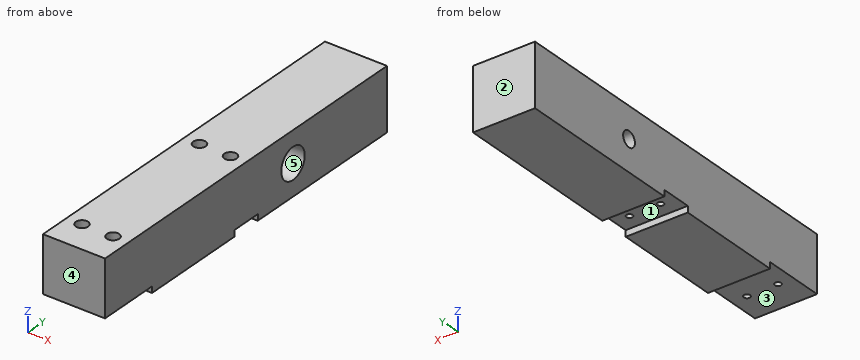
from build123d import *

# Parameters (mm, degrees)
SKETCH1_W           = 20
SKETCH1_H           = 120
SKETCH1_R           = 2.5
BOSS_EXTRUDE2_DEPTH = 20
SKETCH10_R          = 5
CUT_EXTRUDE1_DEPTH  = 10
SKETCH11_R          = 1
CUT_EXTRUDE2_DEPTH  = 21
SKETCH12_R          = 2
CUT_EXTRUDE3_DEPTH  = 5
SKETCH11_3_R        = 1
CUT_EXTRUDE4_DEPTH  = 21
SKETCH14_W          = 20
SKETCH14_H          = 10
SKETCH14_H_2        = 20
CUT_EXTRUDE6_DEPTH  = 2


with BuildPart() as part:
    # Sketch1 → Boss-Extrude2 (new body)
    with BuildSketch(Plane(origin=(0, 0, 0), x_dir=(0, 0, -1), z_dir=(1, 0, 0))):
        with Locations((10, 60)):
            Rectangle(SKETCH1_W, SKETCH1_H)
        with Locations((10, 80)):
            Circle(SKETCH1_R, mode=Mode.SUBTRACT)
    extrude(amount=-BOSS_EXTRUDE2_DEPTH)

    # Sketch10 → Cut-Extrude1 (cut)
    with BuildSketch(Plane(origin=(0, 0, 0), x_dir=(0, 0, -1), z_dir=(1, 0, 0))):
        with Locations((10, 80)):
            Circle(SKETCH10_R)
    extrude(amount=-CUT_EXTRUDE1_DEPTH, mode=Mode.SUBTRACT)

    # Sketch11 → Cut-Extrude2 (cut, through all)
    with BuildSketch(Plane.XY):
        with Locations((-15, 10)):
            Circle(SKETCH11_R)
        with Locations((-5, 10)):
            Circle(SKETCH11_R)
    extrude(amount=-CUT_EXTRUDE2_DEPTH, mode=Mode.SUBTRACT)

    # Sketch12 → Cut-Extrude3 (cut)
    with BuildSketch(Plane.XY):
        with Locations((-15, 10)):
            Circle(SKETCH12_R)
        with Locations((-5, 10)):
            Circle(SKETCH12_R)
        with Locations((-15, 60)):
            Circle(SKETCH12_R)
        with Locations((-5, 60)):
            Circle(SKETCH12_R)
    extrude(amount=-CUT_EXTRUDE3_DEPTH, mode=Mode.SUBTRACT)

    # Sketch11<3> → Cut-Extrude4 (cut, through all)
    with BuildSketch(Plane.XY):
        with Locations((-15, 60)):
            Circle(SKETCH11_3_R)
        with Locations((-5, 60)):
            Circle(SKETCH11_3_R)
    extrude(amount=-CUT_EXTRUDE4_DEPTH, mode=Mode.SUBTRACT)

    # Sketch14 → Cut-Extrude6 (cut)
    with BuildSketch(Plane(origin=(0, 0, -20), x_dir=(-1, 0, 0), z_dir=(0, 0, -1))):
        with Locations((10, 60)):
            Rectangle(SKETCH14_W, SKETCH14_H)
        with Locations((10, 10)):
            Rectangle(SKETCH14_W, SKETCH14_H_2)
    extrude(amount=-CUT_EXTRUDE6_DEPTH, mode=Mode.SUBTRACT)


solid = part.part
Design review of the part built by this model. Coordinates are the model's own, in mm. Face numbers are marked on the shaded views. A direction names the side the tool comes from. Coordinates: 2 decimals unless noted, no trailing zeros. Write each loop counter-clockwise with the first axis right and the second up, starting at its lowest first coordinate (ties: lowest second). Pieces come first, ordered by that corner, then holes. Notation, with made-up numbers: (18, 37.5) - (46, 37.5) arc R8 cw to (46, 42.5) - close; hole circle Ø7 at (84, -11.5). An arc over 180 degrees is marked (long way). Use one line per item in the form item = value.
Q1. For probe 1 along Y at (x, z) = (-5, -3.1); probe 2 along Y at (x, z) = (-5, -9.75); probe 3 along Y at (x, z) = (-3.5, -19), list the stretches that pass through material, from the lowest coordinate up.
Taken from the geometry:
probe_1 = 0 to 8, 12 to 58, 62 to 120
probe_2 = 0 to 9, 11 to 59, 61 to 75.01, 84.99 to 120
probe_3 = 20 to 55, 65 to 120
Q2. The part is to be moulded in two halves that separate along Y. For the marked faces 1, 2 and 3, say which applies: +Y half, -Y half, draft (parallel to the pull), parting line (faces both ways), or undercut.
Taken from the geometry:
face_1 = undercut
face_2 = +Y half
face_3 = draft
Q3. Machinability: for the marked faces 4 and 5, which of the approach directions +Z, -Z, +X, -X, +Y, -Y give a long, thin tool a straight path to every point of the face, cutting with its end or side? Answer none if there is none.
Taken from the geometry:
face_4 = +Z, -Z, +X, -X, -Y
face_5 = +X
Q4. Consider section C-C (z = -10). Write out the cut boundary in (x, y).
Taken from the geometry:
outline = (-20, 0) - (0, 0) - (0, 75) - (-10, 75) - (-10, 77.5) - (-20, 77.5) - close; (-20, 82.5) - (-10, 82.5) - (-10, 85) - (0, 85) - (0, 120) - (-20, 120) - close; hole circle Ø2 at (-15, 10); hole circle Ø2 at (-15, 60); hole circle Ø2 at (-5, 10); hole circle Ø2 at (-5, 60)
Q5. Consider section A-A (x = -15). Write out the cut boundary in (y, z), plus the area to 3 significant figures.
Taken from the geometry:
outline = (0, -18) - (9, -18) - (9, -5) - (8, -5) - (8, 0) - (0, 0) - close; (11, -18) - (20, -18) - (20, -20) - (55, -20) - (55, -18) - (59, -18) - (59, -5) - (58, -5) - (58, 0) - (12, 0) - (12, -5) - (11, -5) - close; (61, -18) - (65, -18) - (65, -20) - (120, -20) - (120, 0) - (62, 0) - (62, -5) - (61, -5) - close; hole circle Ø5 at (80, -10)
area = 2,230 mm^2
Q6. Consider section D-D (y = 80). Write out the cut boundary in (x, z).
Taken from the geometry:
outline = (-20, -20) - (0, -20) - (0, -15) - (-10, -15) - (-10, -12.5) - (-20, -12.5) - close; (-20, -7.5) - (-10, -7.5) - (-10, -5) - (0, -5) - (0, 0) - (-20, 0) - close
Q7. Insertion check: pin 1 Ø3.5 at (x, y) = (-15, 60) entering from -Z; pin 2 Ø1.8 at (x, y) = (-5, 60) entering from +Z; pin 3 Ø3 at (x, y) = (-15, 10) entering from +Z; pin 4 Ø0.6 at (x, z) = (-10.5, -19) entering from -Y. Each pin has a flat end and moves straight along its axis. Give the tip position at first contact, or say it passes through.
Taken from the geometry:
pin_1 = -18
pin_2 = through
pin_3 = -5
pin_4 = 20
Q8. Consider section B-B (y = 10). Write out the cut boundary in (x, z).
Taken from the geometry:
outline = (-20, -18) - (-16, -18) - (-16, -5) - (-17, -5) - (-17, 0) - (-20, 0) - close; (-14, -18) - (-6, -18) - (-6, -5) - (-7, -5) - (-7, 0) - (-13, 0) - (-13, -5) - (-14, -5) - close; (-4, -18) - (0, -18) - (0, 0) - (-3, 0) - (-3, -5) - (-4, -5) - close
